Source: CAD feature listing. Evaluate the final solid. Frame: model axes, mm. A direction names the side the tool comes from. Give positions to 0.01 mm unless a question says otherwise; leave off trailing zeros. Loops run counter-clockwise (first coordinate to the right, second up) from the corner with the lowest first, then second, coordinate; pieces in that order, holes last.
Autodesk Fusion 360 part; units mm, degrees
sketch "Sketch1" plane through (0, 0, 0) normal (0, 1, 0) x (1, 0, 0)
  line L0 (11.7853, -3.8171) -> (86.7853, -3.8171)
  line L1 (91.7853, -8.8171) -> (91.7853, -54.8171)
  line L2 (86.7853, -59.8171) -> (11.7853, -59.8171)
  line L3 (6.7853, -54.8171) -> (6.7853, -8.8171)
  circle A0 centre (10.2853, -7.3171) radius 1.4
  circle A1 centre (10.2853, -56.3171) radius 1.4
  circle A2 centre (68.2853, -7.3171) radius 1.4
  circle A3 centre (68.2853, -56.3171) radius 1.4
  arc A4 (91.7853, -8.8171) -> (86.7853, -3.8171) centre (86.7853, -8.8171) ccw
  arc A5 (86.7853, -59.8171) -> (91.7853, -54.8171) centre (86.7853, -54.8171) ccw
  arc A6 (6.7853, -54.8171) -> (11.7853, -59.8171) centre (11.7853, -54.8171) ccw
  arc A7 (11.7853, -3.8171) -> (6.7853, -8.8171) centre (11.7853, -8.8171) ccw
  dimension "d1" = 85
  dimension "d2" = 56
  dimension "d3" = 58
  dimension "d4" = 2.8
  dimension "d5" = 3.5
  dimension "d6" = 3.5
  dimension "d7" = 49
  dimension "d8" = 5
extrude "Extrude1" add sketch "Sketch1" along normal blind 1.6 makes body 1
copy_body "Body->Comp1" bodies 1 removing the originals makes body 2 in component "PCB"
sketch "Sketch1 (2)" plane through (0, 1.6, 0) normal (0, 1, 0) x (-1, 0, 0) in component "Component"
  circle A0 centre (-68.2853, 56.3171) radius 1.4
  circle A1 centre (-68.2853, 7.3171) radius 1.4
  circle A2 centre (-10.2853, 7.3171) radius 1.4
  circle A3 centre (-10.2853, 56.3171) radius 1.4
  arc A4 (-91.7853, 8.8171) -> (-86.7853, 3.8171) centre (-86.7853, 8.8171) ccw
  line L0 (-86.7853, 3.8171) -> (-11.7853, 3.8171)
  arc A5 (-11.7853, 3.8171) -> (-6.7853, 8.8171) centre (-11.7853, 8.8171) ccw
  line L1 (-6.7853, 8.8171) -> (-6.7853, 54.8171)
  arc A6 (-6.7853, 54.8171) -> (-11.7853, 59.8171) centre (-11.7853, 54.8171) ccw
  line L2 (-11.7853, 59.8171) -> (-86.7853, 59.8171)
  arc A7 (-86.7853, 59.8171) -> (-91.7853, 54.8171) centre (-86.7853, 54.8171) ccw
  line L3 (-91.7853, 54.8171) -> (-91.7853, 8.8171)
  line L4 (-72.7561, 41.6171) -> (-93.8853, 41.6171)
  line L5 (-93.8853, 41.6171) -> (-93.8853, 57.5171)
  line L6 (-93.8853, 57.5171) -> (-72.7561, 57.5171)
  line L7 (-72.7561, 57.5171) -> (-72.7561, 41.6171)
  dimension "d11" = 15.9
  dimension "d12" = 2.3
  dimension "d13" = 87.1
extrude "Extrude1'" add sketch "Sketch1 (2)" along normal blind 13.5 contours A7 L3 L4 L5 L6 | A7 L3 L4 L6 L7 bodies 2 in component "PCB"
sketch "Sketch2" plane through (0, 1.6, 0) normal (0, 1, 0) x (-1, 0, 0)
  line L0 (-72.7561, 41.6171) -> (-91.7853, 41.6171)
  line L1 (-91.7853, 41.6171) -> (-91.7853, 8.8171)
  arc A0 (-91.7853, 8.8171) -> (-86.7853, 3.8171) centre (-86.7853, 8.8171) ccw
  line L2 (-86.7853, 3.8171) -> (-11.7853, 3.8171)
  arc A1 (-11.7853, 3.8171) -> (-6.7853, 8.8171) centre (-11.7853, 8.8171) ccw
  line L3 (-6.7853, 8.8171) -> (-6.7853, 54.8171)
  arc A2 (-6.7853, 54.8171) -> (-11.7853, 59.8171) centre (-11.7853, 54.8171) ccw
  line L4 (-11.7853, 59.8171) -> (-86.7853, 59.8171)
  arc A3 (-86.7853, 59.8171) -> (-90.9936, 57.5171) centre (-86.7853, 54.8171) ccw
  line L5 (-90.9936, 57.5171) -> (-72.7561, 57.5171)
  line L6 (-72.7561, 57.5171) -> (-72.7561, 41.6171)
  circle A4 centre (-68.2853, 56.3171) radius 1.4
  circle A5 centre (-68.2853, 7.3171) radius 1.4
  circle A6 centre (-10.2853, 56.3171) radius 1.4
  circle A7 centre (-10.2853, 7.3171) radius 1.4
  line L7 (-13.5853, 55) -> (-21.0853, 55)
  line L8 (-21.0853, 55) -> (-21.0853, 60.4415)
  line L9 (-21.0853, 60.4415) -> (-13.5853, 60.4415)
  line L10 (-13.5853, 60.4415) -> (-13.5853, 55)
  dimension "d16" = 7.5
  dimension "d17" = 6.8
extrude "Extrude2" add sketch "Sketch2" along normal blind 2.5 contours L4 L8 L9 L10 | L4 L7 L8 L10 bodies 2 in component "PCB"
sketch "Sketch3" plane through (0, 1.6, 0) normal (0, 1, 0) x (-1, 0, 0)
  line L0 (-21.0853, 55) -> (-21.0853, 59.8171)
  line L1 (-21.0853, 59.8171) -> (-86.7853, 59.8171)
  arc A0 (-86.7853, 59.8171) -> (-90.9936, 57.5171) centre (-86.7853, 54.8171) ccw
  line L2 (-90.9936, 57.5171) -> (-72.7561, 57.5171)
  line L3 (-72.7561, 57.5171) -> (-72.7561, 41.6171)
  line L4 (-72.7561, 41.6171) -> (-91.7853, 41.6171)
  line L5 (-91.7853, 41.6171) -> (-91.7853, 8.8171)
  arc A1 (-91.7853, 8.8171) -> (-86.7853, 3.8171) centre (-86.7853, 8.8171) ccw
  line L6 (-86.7853, 3.8171) -> (-11.7853, 3.8171)
  arc A2 (-11.7853, 3.8171) -> (-6.7853, 8.8171) centre (-11.7853, 8.8171) ccw
  line L7 (-6.7853, 8.8171) -> (-6.7853, 54.8171)
  arc A3 (-6.7853, 54.8171) -> (-11.7853, 59.8171) centre (-11.7853, 54.8171) ccw
  line L8 (-11.7853, 59.8171) -> (-13.5853, 59.8171)
  line L9 (-13.5853, 59.8171) -> (-13.5853, 55)
  line L10 (-13.5853, 55) -> (-21.0853, 55)
  circle A4 centre (-68.2853, 56.3171) radius 1.4
  circle A5 centre (-68.2853, 7.3171) radius 1.4
  circle A6 centre (-10.2853, 56.3171) radius 1.4
  circle A7 centre (-10.2853, 7.3171) radius 1.4
  line L11 (-13.3683, 4.6362) -> (-65.3683, 4.6362)
  line L12 (-65.3683, 4.6362) -> (-65.3683, 10.6362)
  line L13 (-65.3683, 10.6362) -> (-13.3683, 10.6362)
  line L14 (-13.3683, 10.6362) -> (-13.3683, 4.6362)
  dimension "d20" = 52
  dimension "d21" = 6
extrude "Extrude3" add sketch "Sketch3" along normal blind 10 contours L11 L12 L13 L14 bodies 2 in component "PCB"
sketch "Sketch4" plane through (0, 1.6, 0) normal (0, 1, 0) x (-1, 0, 0)
  line L0 (-13.3683, 10.6362) -> (-13.3683, 4.6362)
  line L1 (-13.3683, 4.6362) -> (-65.3683, 4.6362)
  line L2 (-65.3683, 4.6362) -> (-65.3683, 10.6362)
  line L3 (-65.3683, 10.6362) -> (-13.3683, 10.6362)
  line L4 (-21.0853, 55) -> (-21.0853, 59.8171)
  line L5 (-21.0853, 59.8171) -> (-86.7853, 59.8171)
  arc A0 (-86.7853, 59.8171) -> (-90.9936, 57.5171) centre (-86.7853, 54.8171) ccw
  line L6 (-90.9936, 57.5171) -> (-72.7561, 57.5171)
  line L7 (-72.7561, 57.5171) -> (-72.7561, 41.6171)
  line L8 (-72.7561, 41.6171) -> (-91.7853, 41.6171)
  line L9 (-91.7853, 41.6171) -> (-91.7853, 8.8171)
  arc A1 (-91.7853, 8.8171) -> (-86.7853, 3.8171) centre (-86.7853, 8.8171) ccw
  line L10 (-86.7853, 3.8171) -> (-11.7853, 3.8171)
  arc A2 (-11.7853, 3.8171) -> (-6.7853, 8.8171) centre (-11.7853, 8.8171) ccw
  line L11 (-6.7853, 8.8171) -> (-6.7853, 54.8171)
  arc A3 (-6.7853, 54.8171) -> (-11.7853, 59.8171) centre (-11.7853, 54.8171) ccw
  line L12 (-11.7853, 59.8171) -> (-13.5853, 59.8171)
  line L13 (-13.5853, 59.8171) -> (-13.5853, 55)
  line L14 (-13.5853, 55) -> (-21.0853, 55)
  circle A4 centre (-68.2853, 56.3171) radius 1.4
  circle A5 centre (-68.2853, 7.3171) radius 1.4
  circle A6 centre (-10.2853, 56.3171) radius 1.4
  circle A7 centre (-10.2853, 7.3171) radius 1.4
  line L15 (-30.1471, 21.6994) -> (-46.1471, 21.6994)
  line L16 (-46.1471, 21.6994) -> (-46.1471, 37.6994)
  line L17 (-46.1471, 37.6994) -> (-30.1471, 37.6994)
  line L18 (-30.1471, 37.6994) -> (-30.1471, 21.6994)
  dimension "d24" = 16
  dimension "d25" = 16
extrude "Extrude4" add sketch "Sketch4" along normal blind 2 contours L15 L16 L17 L18 bodies 2 in component "PCB"
sketch "Sketch5" plane through (0, 1.6, 0) normal (0, 1, 0) x (-1, 0, 0)
  line L0 (-30.1471, 37.6994) -> (-30.1471, 21.6994)
  line L1 (-30.1471, 21.6994) -> (-46.1471, 21.6994)
  line L2 (-46.1471, 21.6994) -> (-46.1471, 37.6994)
  line L3 (-46.1471, 37.6994) -> (-30.1471, 37.6994)
  line L4 (-13.3683, 10.6362) -> (-13.3683, 4.6362)
  line L5 (-13.3683, 4.6362) -> (-65.3683, 4.6362)
  line L6 (-65.3683, 4.6362) -> (-65.3683, 10.6362)
  line L7 (-65.3683, 10.6362) -> (-13.3683, 10.6362)
  line L8 (-21.0853, 55) -> (-21.0853, 59.8171)
  line L9 (-21.0853, 59.8171) -> (-86.7853, 59.8171)
  arc A0 (-86.7853, 59.8171) -> (-90.9936, 57.5171) centre (-86.7853, 54.8171) ccw
  line L10 (-90.9936, 57.5171) -> (-72.7561, 57.5171)
  line L11 (-72.7561, 57.5171) -> (-72.7561, 41.6171)
  line L12 (-72.7561, 41.6171) -> (-91.7853, 41.6171)
  line L13 (-91.7853, 41.6171) -> (-91.7853, 8.8171)
  arc A1 (-91.7853, 8.8171) -> (-86.7853, 3.8171) centre (-86.7853, 8.8171) ccw
  line L14 (-86.7853, 3.8171) -> (-11.7853, 3.8171)
  arc A2 (-11.7853, 3.8171) -> (-6.7853, 8.8171) centre (-11.7853, 8.8171) ccw
  line L15 (-6.7853, 8.8171) -> (-6.7853, 54.8171)
  arc A3 (-6.7853, 54.8171) -> (-11.7853, 59.8171) centre (-11.7853, 54.8171) ccw
  line L16 (-11.7853, 59.8171) -> (-13.5853, 59.8171)
  line L17 (-13.5853, 59.8171) -> (-13.5853, 55)
  line L18 (-13.5853, 55) -> (-21.0853, 55)
  circle A4 centre (-68.2853, 56.3171) radius 1.4
  circle A5 centre (-68.2853, 7.3171) radius 1.4
  circle A6 centre (-10.2853, 56.3171) radius 1.4
  circle A7 centre (-10.2853, 7.3171) radius 1.4
  line L19 (-76.4643, 24.3171) -> (-93.7853, 24.3171)
  line L20 (-93.7853, 24.3171) -> (-93.7853, 37.4171)
  line L21 (-93.7853, 37.4171) -> (-76.4643, 37.4171)
  line L22 (-76.4643, 37.4171) -> (-76.4643, 24.3171)
  line L23 (-76.2496, 19.4171) -> (-93.7853, 19.4171)
  line L24 (-93.7853, 19.4171) -> (-93.7853, 6.3171)
  line L25 (-93.7853, 6.3171) -> (-76.2496, 6.3171)
  line L26 (-76.2496, 6.3171) -> (-76.2496, 19.4171)
  dimension "d28" = 13.1
  dimension "d29" = 4.2
  dimension "d30" = 2
  dimension "d31" = 13.1
  dimension "d32" = 4.9
extrude "Extrude5" add sketch "Sketch5" along normal blind 18.8 contours L13 L19 L21 L22 | L13 L19 L20 L21 | L13 A1 L23 L24 L25 | L13 A1 L23 L25 L26 bodies 2 in component "PCB"
component "Component" placed x (1, 0, 0) y (0, 1, 0) z (0, 0, 1) at (0, 0, 0)
component "PCB" placed x (1, 0, 0) y (0, 1, 0) z (0, 0, 1) at (0, 0, 0)
1) Contact query for flat-ended pins moving along their axis: P1, Ø2, axis at x = 41, z = 24.5, coming from the +Y side; P2, Ø4.5, axis at x = 17, z = 58.5, coming from the +Y side; P3, Ø4, axis at x = 87, y = 9, coming from the -Z side. Output: stop coordinate, or through.
Checks:
P1: stops at y = 3.6
P2: stops at y = 4.1
P3: stops at z = 6.32
2) Reachability of faces 1 (the flat face through (93.785, 11, 13)), 2 (the flat face through (83, 15.1, 50)), 3 (the flat face through (40, 11.6, 8)), 4 (the flat face through (85, 11, 19.417)) from +Z, -Z, +X, -X, +Y, -Y: full face, straight path, thin tool, end or side. Return the list, or none.
Checks:
face 1: -Z, +X, +Y, -Y
face 2: +Z, +X, -X, +Y
face 3: +Z, -Z, -X, +Y
face 4: +X, -X, +Y
3) Ray query, probe 1 along Z at (x, y) = (88.5, 16.25); probe 2 along X at (y, z) = (11.5, 7.5); probe 3 along X at (y, z) = (9.25, 28.5). Return the intervals inside material, ascending.
Checks:
probe 1: z = 6.32 to 19.42, 24.32 to 37.42
probe 2: x = 13.37 to 65.37, 76.25 to 93.79
probe 3: x = 76.46 to 93.79
4) Cut plane B-B (y = 5.75). Return loops of the section in (x, z), and give its area (3 significant figures).
Checks:
outline: (13.37, 4.64) - (65.37, 4.64) - (65.37, 10.64) - (13.37, 10.64) - close; (72.76, 41.62) - (93.89, 41.62) - (93.89, 57.52) - (72.76, 57.52) - close; (76.25, 6.32) - (93.79, 6.32) - (93.79, 19.42) - (76.25, 19.42) - close; (76.46, 24.32) - (93.79, 24.32) - (93.79, 37.42) - (76.46, 37.42) - close
area: 1,100 mm2
5) Pull-direction query (X, two-part tool) for faces 5 (the flat face through (93.885, 8, 49)), 6 (the cylindrical face through (8.21, 0.79, 5.32)), 7 (the cylindrical face through (69.62, 0.79, 56.74)); classes: released by +X, released by -X, zero draft, split by the parting line, or undercut.
Checks:
face 5: released by +X
face 6: released by -X
face 7: undercut
6) Cut plane A-A (y = 18.5). Return loops of the section in (x, z), and give its area (3 significant figures).
Checks:
outline: (76.25, 6.32) - (93.79, 6.32) - (93.79, 19.42) - (76.25, 19.42) - close; (76.46, 24.32) - (93.79, 24.32) - (93.79, 37.42) - (76.46, 37.42) - close
area: 457 mm2
7) Cut plane C-C (x = 38). Return loops of the section in (y, z).
Checks:
outline: (0, 3.82) - (1.6, 3.82) - (1.6, 4.64) - (11.6, 4.64) - (11.6, 10.64) - (1.6, 10.64) - (1.6, 21.7) - (3.6, 21.7) - (3.6, 37.7) - (1.6, 37.7) - (1.6, 59.82) - (0, 59.82) - close
8) Cut plane D-D (z = 35). Return loops of the section in (x, y), and give its area (3 significant figures).
Checks:
outline: (6.79, 0) - (91.79, 0) - (91.79, 1.6) - (93.79, 1.6) - (93.79, 20.4) - (76.46, 20.4) - (76.46, 1.6) - (46.15, 1.6) - (46.15, 3.6) - (30.15, 3.6) - (30.15, 1.6) - (6.79, 1.6) - close
area: 494 mm2
